```python
from build123d import *

# Parameters (mm, degrees)
SKETCH1_W                        = 98
SKETCH1_H                        = 60
BOSS_EXTRUDE1_DEPTH              = 11
SKETCH2_W                        = 9.4
SKETCH2_H                        = 10
CUT_EXTRUDE1_DEPTH               = 99
SKETCH3_W                        = 9.4
SKETCH3_H                        = 10
CUT_EXTRUDE2_DEPTH               = 99
SKETCH4_W                        = 3.935514966
SKETCH4_H                        = 1.073322306
BOSS_EXTRUDE2_DEPTH              = 3
SKETCH5_W                        = 3.015
SKETCH5_H                        = 1.118767377
BOSS_EXTRUDE3_DEPTH              = 3
SKETCH6_W                        = 76
SKETCH6_H                        = 25.2
CUT_EXTRUDE3_DEPTH               = 0.5
F_2_5_2_5_DIAMETER_HOLE1_D       = 2.5
F_2_5_2_5_DIAMETER_HOLE1_DEPTH   = 11
F_0_95_0_95_DIAMETER_HOLE1_D     = 0.95
F_0_95_0_95_DIAMETER_HOLE1_DEPTH = 11


with BuildPart() as part:
    # Sketch1 → Boss-Extrude1 (new body)
    with BuildSketch(Plane.XY.offset(11)):
        Rectangle(SKETCH1_W, SKETCH1_H)
    extrude(amount=-BOSS_EXTRUDE1_DEPTH)

    # Sketch2 → Cut-Extrude1 (cut, through all)
    with BuildSketch(Plane(origin=(49, 0, 0), x_dir=(0, 0, -1), z_dir=(1, 0, 0))):
        with Locations((-6.3, -25)):
            Rectangle(SKETCH2_W, SKETCH2_H)
    extrude(amount=-CUT_EXTRUDE1_DEPTH, mode=Mode.SUBTRACT)

    # Sketch3 → Cut-Extrude2 (cut, through all)
    with BuildSketch(Plane(origin=(49, 0, 0), x_dir=(0, 0, -1), z_dir=(1, 0, 0))):
        with Locations((-6.3, 25)):
            Rectangle(SKETCH3_W, SKETCH3_H)
    extrude(amount=-CUT_EXTRUDE2_DEPTH, mode=Mode.SUBTRACT)

    # Sketch4 → Boss-Extrude2 (add)
    with BuildSketch(Plane(origin=(0, 0, 0), x_dir=(-1, 0, 0), z_dir=(0, 0, -1))):
        with Locations((-34.644135617, 16.964786449)):
            Rectangle(SKETCH4_W, SKETCH4_H)
    extrude(amount=BOSS_EXTRUDE2_DEPTH)

    # Sketch5 → Boss-Extrude3 (add)
    with BuildSketch(Plane(origin=(0, 0, 0), x_dir=(-1, 0, 0), z_dir=(0, 0, -1))):
        with Locations((27.8075, -21.700286291)):
            Rectangle(SKETCH5_W, SKETCH5_H)
    extrude(amount=BOSS_EXTRUDE3_DEPTH)

    # Sketch6 → Cut-Extrude3 (cut)
    with BuildSketch(Plane.XY.offset(11)):
        Rectangle(SKETCH6_W, SKETCH6_H)
    extrude(amount=-CUT_EXTRUDE3_DEPTH, mode=Mode.SUBTRACT)

    # Ø2.5 (2.5) Diameter Hole1
    with Locations(Plane(origin=(0, 0, 0), x_dir=(-1, 0, 0), z_dir=(0, 0, -1))):
        with Locations((46.5, -27.5), (-46.5, -27.5), (-46.5, 27.5), (46.5, 27.5)):
            Hole(F_2_5_2_5_DIAMETER_HOLE1_D / 2, depth=F_2_5_2_5_DIAMETER_HOLE1_DEPTH)

    # Ø0.95 (0.95) Diameter Hole1
    with Locations(Plane(origin=(0, 0, 0), x_dir=(-1, 0, 0), z_dir=(0, 0, -1))):
        with Locations((0.9, 27), (3.44, 27), (5.98, 27), (8.52, 27), (11.06, 27), (13.6, 27), (16.14, 27), (18.68, 27), (21.22, 27), (23.76, 27), (26.3, 27), (28.84, 27), (31.38, 27), (33.92, 27), (36.46, 27), (39, 27)):
            Hole(F_0_95_0_95_DIAMETER_HOLE1_D / 2, depth=F_0_95_0_95_DIAMETER_HOLE1_DEPTH)


solid = part.part
```
Geometry check sheet. Reference: the model listing, model coordinates, mm. A direction names the side the tool comes from. Give positions to 0.01 mm unless a question says otherwise; leave off trailing zeros. Write each loop counter-clockwise with the first axis right and the second up, starting at its lowest first coordinate (ties: lowest second). Pieces come first, ordered by that corner, then holes.
1) Release check for a two-part mould opening along X. For faces 6 (the flat face through (-1, 0, 0)), 7 (the flat face through (-1, 0, 10.5)), 8 (the flat face through (-49, 0, 6)) record: pulls with the +X half, pulls with the -X half, needs draft (parallel to the pull), parting line crosses it, or undercut.
2) Section check B-B, the plane z = -1.75. Record the boundary of the cut face in (x, y) (3 decimals), and give its area (3 significant figures).
3) Gauge pin test, flat ends, axial feed: pin 1 (1.5 mm diameter, centred on x = -28, z = -2, fed in from +Y); pin 2 (12 mm diameter, centred on x = -15.5, y = 3, fed in from -Z); pin 3 (4 mm diameter, centred on x = -32, z = 4, fed in from +Y). Record the tip position at first contact, or that the pin passes through.
4) Material ranges on L1, parallel to Y at x = 46.5, z = 0.75; L2, parallel to Y at x = -36.46, z = 0.45 (3 decimals); L3, parallel to Z at x = 18, y = -26, recorded low to high.
5) Access from +Z, -Z, +X, -X, +Y, -Y to the whole of each face (thin tool, end or side, straight path). Record for faces 1 (the flat face through (-1, 14, 11)), 2 (the flat face through (1, -20, 6)), 3 (the flat face through (1, 20, 6)), 4 (the flat face through (-28, -22.26, -1)), 5 (the flat face through (-28, -21.141, -1)).
6) Section check A-A, the plane x = -46.5. Record the boundary of the cut face in (y, z), and give its area (3 significant figures).
7) Section check C-C, the plane y = 6.5. Record the boundary of the cut face in (x, z).
8) Section check D-D, the plane x = 6. Record the boundary of the cut face in (y, z).
Computed:
1. face 6: needs draft
1. face 7: undercut
1. face 8: pulls with the -X half
2. outline: (-29.315, -22.26) - (-26.3, -22.26) - (-26.3, -21.141) - (-29.315, -21.141) - close; (32.676, 16.428) - (36.612, 16.428) - (36.612, 17.501) - (32.676, 17.501) - close
2. area: 7.60 mm2
3. pin 1: stops at y = -21.14
3. pin 2: stops at z = 0
3. pin 3: stops at y = 20
4. L1: y = -30 to -28.75, -26.25 to 26.25, 28.75 to 30
4. L2: y = -30 to 26.525, 27.475 to 30
4. L3: z = 0 to 1.6
5. face 1: +Z, +X, -X, +Y, -Y
5. face 2: +Z, +X, -X, -Y
5. face 3: +Z, +X, -X, +Y
5. face 4: -Z, +X, -X, -Y
5. face 5: -Z, +X, -X, +Y
6. outline: (-30, 0) - (-28.75, 0) - (-28.75, 1.6) - (-30, 1.6) - close; (-26.25, 0) - (26.25, 0) - (26.25, 1.6) - (20, 1.6) - (20, 11) - (-20, 11) - (-20, 1.6) - (-26.25, 1.6) - close; (28.75, 0) - (30, 0) - (30, 1.6) - (28.75, 1.6) - close
6. area: 464 mm2
7. outline: (-49, 0) - (49, 0) - (49, 11) - (38, 11) - (38, 10.5) - (-38, 10.5) - (-38, 11) - (-49, 11) - close
8. outline: (-30, 0) - (30, 0) - (30, 1.6) - (20, 1.6) - (20, 11) - (12.6, 11) - (12.6, 10.5) - (-12.6, 10.5) - (-12.6, 11) - (-20, 11) - (-20, 1.6) - (-30, 1.6) - close
